Autodesk Inventor part; units mm, degrees
ref_plane "YZ Plane" through (0, 0, 0) normal (1, 0, 0) x (0, 1, 0)
ref_plane "XZ Plane" through (0, 0, 0) normal (0, 1, 0) x (-1, 0, 0)
ref_plane "XY Plane" through (0, 0, 0) normal (0, 0, 1) x (1, 0, 0)
sketch "Sketch1" plane through (0, 0, 0) normal (0, 0, 1) x (1, 0, 0)
  line L0 (-15.3704, -21.125) -> (-12.625, -21.125)
  line L1 (0, 21.125) -> (-15.3704, 21.125)
  line L2 (-21.125, 15.3704) -> (-21.125, -15.3704)
  arc A0 (-15.3704, 21.125) -> (-21.125, 15.3704) centre (0, 0) ccw
  arc A1 (-21.125, -15.3704) -> (-15.3704, -21.125) centre (0, 0) ccw
  line L3 (0, 21.125) -> (0, 24.125)
  line L4 (0, 24.125) -> (-16.3172, 24.125)
  arc A2 (-16.3172, 24.125) -> (-24.125, 16.3172) centre (0, 0) ccw
  line L5 (-24.125, 16.3172) -> (-24.125, -16.3172)
  arc A3 (-24.125, -16.3172) -> (-16.3172, -24.125) centre (0, 0) ccw
  line L6 (-16.3172, -24.125) -> (-12.625, -24.125)
  arc A4 (-12.625, -24.125) -> (-12.625, -21.125) centre (-12.625, -22.625) ccw
  line L7 (-26.625, 42.6643) -> (-26.625, 23.9143)
  line L8 (-26.625, 23.9143) -> (-24.125, 23.9143)
  line L9 (-24.125, 23.9143) -> (-24.125, 20.7893)
  arc A5 (-30.9534, 17.9609) -> (-24.125, 20.7893) centre (-28.125, 20.7893) ccw
  arc A6 (-30.9534, 17.9609) -> (-32.3676, 16.5467) centre (-31.6605, 17.2538) ccw
  arc A7 (-32.3676, 16.5467) -> (-22.125, 20.7893) centre (-28.125, 20.7893) ccw
  line L10 (-31.6605, 17.2538) -> (-28.125, 20.7893) construction
  line L11 (-26.625, 42.6643) -> (-22.125, 42.6643)
  line L12 (-22.125, 42.6643) -> (-22.125, 20.7893)
  line L13 (-16.3172, 24.125) -> (-22.125, 24.125)
  line L14 (-22.125, 42.6643) -> (-22.125, 64.5393)
  line L15 (-22.125, 64.5393) -> (16.3172, 24.125)
  line L16 (16.3172, 24.125) -> (0, 24.125)
  point P0 (-22.6762, 18.2771)
  dimension "d2" = 42.25
  dimension "d3" = 26.125
  dimension "d5" = 21.125
  dimension "d6" = 3
  dimension "d7" = 3
  dimension "d8" = 3
  dimension "d9" = 3
  dimension "d10" = 3
  dimension "d11" = 10
  dimension "d12" = 45
  dimension "d13" = 18.75
  dimension "d14" = 25.875
  dimension "d15" = 4
  dimension "d17" = 2
  dimension "d18" = 2.5
  dimension "d21" = 21.125
  dimension "d33" = 16.3172
  dimension "d34" = 16.3172
  dimension "d35" = 21.875
  dimension "d36" = 21.875
extrude "Extrusion1" add sketch "Sketch1" along normal blind 14.25 contours L0 A4 L6 A3 L5 A7 A2 L4 L3 L1 A0 L2 A1 | A2 A7
mirror "Mirror1" about plane through (0, 0, 0) normal (1, 0, 0)
extrude "Extrusion2" add sketch "Sketch1" along normal blind 14.25 separate body contours A7 A6 A5 L9 L8 L7 L11 L12 A2 | A2 A7
chamfer "Chamfer1" distance 1 angle 45 1 edges at (-26.625, 23.9143, 7.125)
mirror "Mirror2" about plane through (-22.125, 42.6643, 0) normal (0, 1, 0) bodies 2
extrude "Extrusion3" add sketch "Sketch1" along normal blind 1 contours L4 L13 L12 L14 L15 L16 bodies 2
extrude "Extrusion4" add sketch "Sketch1" along normal blind 14.25 contours A7 L12 L13 A2 bodies 2
combine bodies "Combine1" operation type add bodies to combine 2 1
fillet "Fillet1" radius 5 1 edges at (-22.125, 24.125, 7.625)
equation "\"d2\" = d0"
equation "\"d7\" = d6"
equation "\"d8\" = d6"
equation "\"d9\" = d6"
equation "\"d10\" = d6"
equation "\"d34\" = d33"
equation "\"d35\" = d36"
equation "\"d22\" = d19"
equation "\"d31\" = d19"
properties part number "Daiso Phone Printer Adapter"
The listing builds one solid part. Answer for the finished solid, in the listing's coordinates (mm). A direction names the side the tool comes from. Give positions to 0.01 mm unless a question says otherwise; leave off trailing zeros. Order: outer loops, then holes, each group sorted by start corner. A loop starts at its lowest first (then second) coordinate and runs counter-clockwise, first axis right, second up.
1) Determine the mould class of faces 4 (the face through (-25.92, 70.12, 7.03)), 5 (the face through (0, 24.125, 8)), 6 (the face through (24.125, 0, 7)), 7 (the face through (-28.23, 14.79, 7.03)) for opening direction X: pulls with the +X half, pulls with the -X half, needs draft (parallel to the pull), parting line crosses it, or undercut.
Reported:
face 4: parting line crosses it
face 5: needs draft
face 6: pulls with the +X half
face 7: undercut
2) Find section A-A on y = -9. Write down the section's boundary in (x, z) (3 decimals), then the cut area to 3 significant figures.
Reported:
outline: (-24.125, 0) - (-21.125, 0) - (-21.125, 14.25) - (-24.125, 14.25) - close; (21.125, 0) - (24.125, 0) - (24.125, 14.25) - (21.125, 14.25) - close
area: 85.5 mm2
3) Find section D-D on x = -2. Write down the section's boundary in (y, z) (3 decimals).
Reported:
outline: (21.125, 0) - (43.382, 0) - (43.382, 1) - (24.125, 1) - (24.125, 14.25) - (21.125, 14.25) - close
4) Consider line 1 along Y through (x, z) = (-13, 11.75) (3 decimals); line 2 along Y through (x, z) = (4, 10.25) (3 decimals). Determine where each line is inside the solid, lowest interval first.
Reported:
line 1: y = -24.125 to -21.125, 21.125 to 24.125
line 2: y = 21.125 to 24.125
5) Find section B-B on x = 19. Write down the section's boundary in (y, z).
Reported:
outline: (-22.07, 0) - (-17.93, 0) - (-17.93, 14.25) - (-22.07, 14.25) - close; (17.93, 0) - (22.07, 0) - (22.07, 14.25) - (17.93, 14.25) - close
6) For faces 1 (the face through (-24.125, 22, 7)), 2 (the face through (-20.7, 25.63, 7.72)), 3 (the face through (-18.433, -18.514, 7.025)), determine the directions among +Z, -Z, +X, -X, +Y, -Y from which every point of the face is accessible in a straight line to the end or side of a thin tool.
Reported:
face 1: +Z, -Z, -X
face 2: +Z, +X, +Y
face 3: +Z, -Z
7) Given P1, Ø6, axis at x = 11, z = 9, coming from the -Y side (3 decimals); P2, Ø0.8, axis at x = -25, z = 8.5, coming from the -Y side; P3, Ø0.8, axis at x = -24.5, z = 8.5, coming from the +Y side; P4, Ø4.5, axis at x = 7.5, z = 4, coming from the -Y side (3 decimals), each flat-ended and moving along its own axis, determine where each tip first touches the part or whether it passes through.
Reported:
P1: stops at y = -24.125
P2: stops at y = 15.44
P3: stops at y = 69.6
P4: stops at y = 21.125
